```python
from build123d import *

# Parameters (mm, degrees)
SKETCH1_W                                       = 254
SKETCH1_H                                       = 76.2
BOSS_EXTRUDE1_DEPTH                             = 12.7
F_1_4_CLEARANCE_HOLE1_D                         = 6.5278
CHAMFER1_SIZE                                   = 6.35
CSK_FOR_M5_FLAT_HEAD_MACHINE_SCREW1_D           = 5.8
CSK_FOR_M5_FLAT_HEAD_MACHINE_SCREW1_CSINK_D     = 10.4
CSK_FOR_M5_FLAT_HEAD_MACHINE_SCREW1_CSINK_ANGLE = 90


with BuildPart() as part:
    # Sketch1 → Boss-Extrude1 (new body)
    with BuildSketch(Plane.XY):
        Rectangle(SKETCH1_W, SKETCH1_H)
    extrude(amount=BOSS_EXTRUDE1_DEPTH)

    # 1/4 Clearance Hole1 (through all)
    with Locations(Plane.XY.offset(12.7)):
        with Locations((38.1, 14.2875), (-117.475, -28.575), (-117.475, 28.575), (117.475, -28.575), (117.475, 28.575), (-38.1, 14.2875), (0, -14.2875)):
            Hole(F_1_4_CLEARANCE_HOLE1_D / 2)

    # Chamfer1
    chamfer1_edges = [part.edges().sort_by_distance(p)[0] for p in [
        (-127, 38.1, 6.35),
        (127, 38.1, 6.35),
        (127, -38.1, 6.35),
        (-127, -38.1, 6.35),
    ]]
    chamfer(chamfer1_edges, length=CHAMFER1_SIZE)

    # CSK for M5 Flat Head Machine Screw1 (through all)
    with Locations(Plane(origin=(0, 0, 0), x_dir=(-1, 0, 0), z_dir=(0, 0, -1))):
        with Locations((-81.25, -25), (-81.25, 25), (83.05, 25), (83.05, -25), (-84.25, 0), (84.25, 0)):
            CounterSinkHole(CSK_FOR_M5_FLAT_HEAD_MACHINE_SCREW1_D / 2, CSK_FOR_M5_FLAT_HEAD_MACHINE_SCREW1_CSINK_D / 2, counter_sink_angle=CSK_FOR_M5_FLAT_HEAD_MACHINE_SCREW1_CSINK_ANGLE)


solid = part.part
```
Design review of the part built by this model. Coordinates are the model's own, in mm. Coordinates: 2 decimals unless noted, no trailing zeros. Loops run counter-clockwise (first coordinate to the right, second up) from the corner with the lowest first, then second, coordinate; pieces in that order, holes last.
Q1. The part is to be moulded in two halves that separate along Y. For faces 1 (the face through (81.353, 0.128, 7.573)), 2 (the face through (127, 0, 6)), 3 (the face through (-120.49, 27.32, 6.26)), 4 (the face through (-123.78, 34.97, 6.26)), say which applies: +Y half, -Y half, draft (parallel to the pull), parting line (faces both ways), or undercut.
Reported:
face 1: undercut
face 2: draft
face 3: undercut
face 4: +Y half
Q2. We need section A-A on x = 38.1. State the section outline as (y, z) points, and give its area (3 significant figures).
Reported:
outline: (-38.1, 0) - (11.02, 0) - (11.02, 12.7) - (-38.1, 12.7) - close; (17.55, 0) - (38.1, 0) - (38.1, 12.7) - (17.55, 12.7) - close
area: 885 mm2
Q3. To check wall thickness, follow line 1 (Y direction, x = 81.25, z = 8.75); line 2 (X direction, y = -28, z = 10.5); line 3 (X direction, y = 24.5, z = 11). State the ranges of each line that lie inside material, in increasing order.
Reported:
line 1: y = -38.1 to -27.9, -22.1 to 22.1, 27.9 to 38.1
line 2: x = -127 to -120.69, -114.26 to 114.26, 120.69 to 127
line 3: x = -127 to -85.91, -80.19 to 78.39, 84.11 to 127
Q4. For pin 1 (6.5 mm diameter, centred on x = -83.05, y = -25, fed in from -Z), flat-tipped, find the tip position at first contact; note if it passes through.
Reported:
pin 1: stops at z = 1.95
Q5. We need section B-B on z = 6.75. State how many separate pieces and enclosed holes the cut face has, and give its area (3 significant figures).
Reported:
separate pieces: 1
enclosed holes: 13
area: 18,900 mm2
